Verification items for this drawing (mm, ordinates from the low corner). Coordinates: 2 decimals unless noted, no trailing zeros. Write each loop counter-clockwise with the first axis right and the second up, starting at its lowest first coordinate (ties: lowest second). Pieces come first, ordered by that corner, then holes.
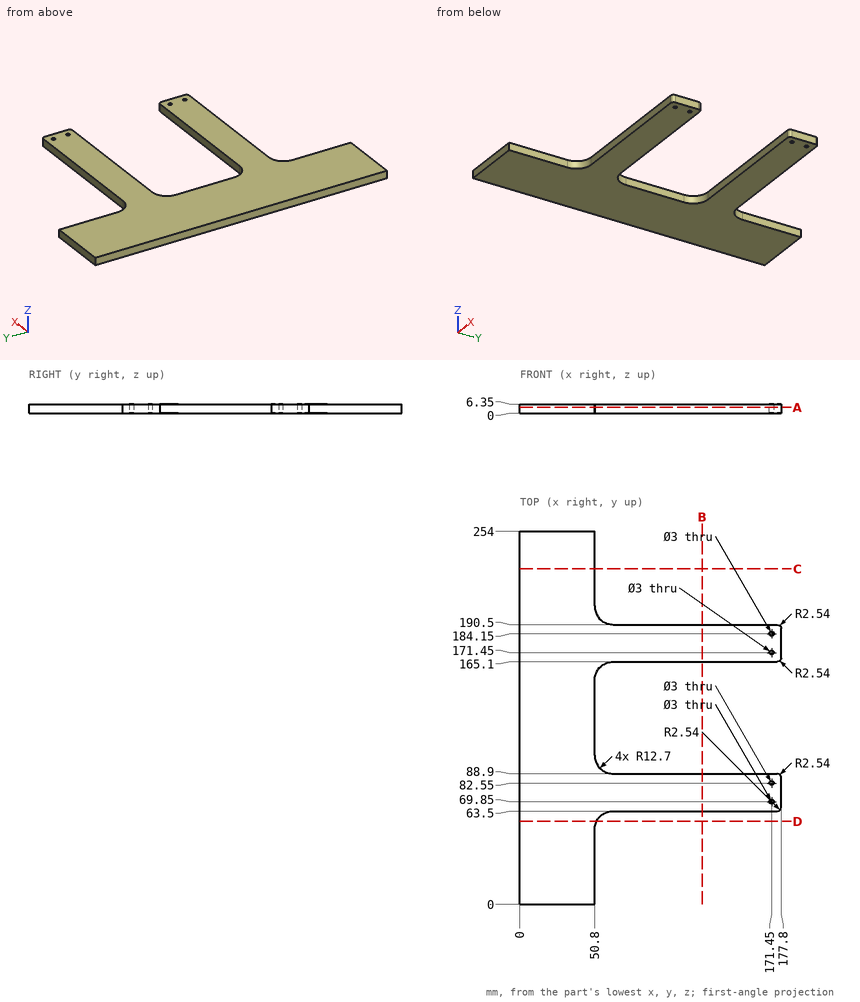
1. Thickness scan on line 1 along Y through (x, z) = (171.45, 2.75); line 2 along X through (y, z) = (184.5, 1.5); line 3 along Y through (x, z) = (130.5, 3.25). Record the ranges inside material, lowest first.
Computed values:
line 1: y = 63.5 to 68.35, 71.35 to 81.05, 84.05 to 88.9, 165.1 to 169.95, 172.95 to 182.65, 185.65 to 190.5
line 2: x = 0 to 169.99, 172.91 to 177.8
line 3: y = 63.5 to 88.9, 165.1 to 190.5
2. Sectioned sample at D-D, the plane y = 56.5. Record the boundary of the cut face in (x, z), and give its area (3 significant figures).
Computed values:
outline: (0, 0) - (52.15, 0) - (52.15, 6.35) - (0, 6.35) - close
area: 331 mm2
3. Gauge pin test, flat ends, axial feed: pin 1 Ø1.9 at (x, z) = (121, 2.5) entering from -Y; pin 2 Ø3 at (y, z) = (238.5, 3.5) entering from +X. Record the tip position at first contact, or that the pin passes through.
Computed values:
pin 1: stops at y = 63.5
pin 2: stops at x = 50.8
4. Sectioned sample at A-A, the plane z = 4. Record the boundary of the cut face in (x, y).
Computed values:
outline: (0, 0) - (50.8, 0) - (50.8, 50.8) arc R12.7 cw to (63.5, 63.5) - (175.26, 63.5) arc R2.54 ccw to (177.8, 66.04) - (177.8, 86.36) arc R2.54 ccw to (175.26, 88.9) - (63.5, 88.9) arc R12.7 cw to (50.8, 101.6) - (50.8, 152.4) arc R12.7 cw to (63.5, 165.1) - (175.26, 165.1) arc R2.54 ccw to (177.8, 167.64) - (177.8, 187.96) arc R2.54 ccw to (175.26, 190.5) - (63.5, 190.5) arc R12.7 cw to (50.8, 203.2) - (50.8, 254) - (0, 254) - close; hole circle Ø3 at (171.45, 69.85); hole circle Ø3 at (171.45, 82.55); hole circle Ø3 at (171.45, 171.45); hole circle Ø3 at (171.45, 184.15)
5. Sectioned sample at B-B, the plane x = 124. Record the boundary of the cut face in (y, z), and give its area (3 significant figures).
Computed values:
outline: (63.5, 0) - (88.9, 0) - (88.9, 6.35) - (63.5, 6.35) - close; (165.1, 0) - (190.5, 0) - (190.5, 6.35) - (165.1, 6.35) - close
area: 323 mm2
6. Sectioned sample at C-C, the plane y = 228.5. Record the boundary of the cut face in (x, z).
Computed values:
outline: (0, 0) - (50.8, 0) - (50.8, 6.35) - (0, 6.35) - close
